For this review, take the finished solid that the model builds, in its own axes (mm). Face numbers are marked on the shaded views. A direction names the side the tool comes from. Give positions to 0.01 mm unless a question says otherwise; leave off trailing zeros. Order: outer loops, then holes, each group sorted by start corner. A loop starts at its lowest first (then second) coordinate and runs counter-clockwise, first axis right, second up. Notation, with made-up numbers: M -20,63 L 24,63 A26 ccw 24,81 Z; hole C 88,6 d9. An arc over 180 degrees is marked long. Answer as CSV lines item,"result". Start each with the question number.
1. Machinability: for the marked faces 1 and 2, which of the approach directions +Z, -Z, +X, -X, +Y, -Y give a long, thin tool a straight path to every point of the face, cutting with its end or side? Answer none if there is none.
2. For line 1 along Y through (x, z) = (36.75, 0); line 2 along X through (y, z) = (-6.75, 8.5); line 3 along Z through (x, y) = (28.5, 0.75), list the stretches that pass through material, from the lowest coordinate up.
3. Mouldability with a two-part tool opening along Y and no side actions: class the marked faces 3, 4 and 5 as pulls with the +Y half, pulls with the -Y half, needs draft (parallel to the pull), parting line crosses it, or undercut.
4. We need section D-D, the plane x = 1. Give the boundary of the cut face in (y, z), and give its area (3 significant figures).
5. We need section A-A, the plane y = 0. Give the boundary of the cut face in (x, z).
6. Clearance check with flat-ended pins moving along their axes: P1, Ø4, axis at x = 28.5, z = 7.5, coming from the -Y side; P2, Ø1.5, axis at x = -31.5, y = -3, coming from the +Z side; P3, Ø8, axis at x = -27.5, y = -5.5, coming from the +Z side. State where each tip first meets the part, or that it passes through.
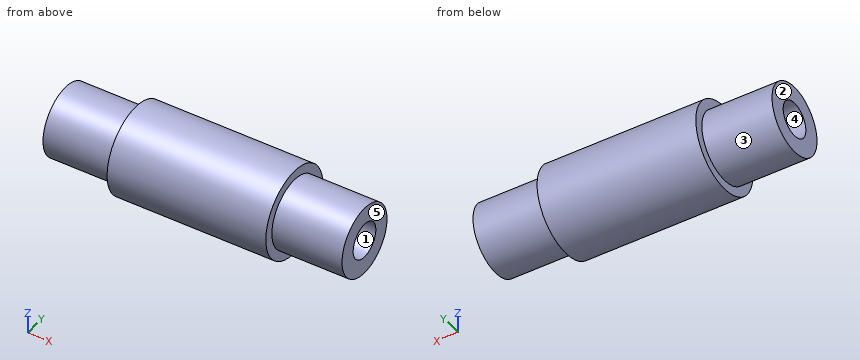
from build123d import *

# Parameters (mm, degrees)
SOCKET_1_SKETCH_W = 17.8
SOCKET_1_SKETCH_H = 4.7625
SOCKET_2_SKETCH_W = 17.8
SOCKET_2_SKETCH_H = 4.7625


with BuildPart() as part:
    # Filter_F2_T6 Sketch → Filter_F2_T6 (revolve)
    with BuildSketch(Plane.XY, mode=Mode.PRIVATE) as filter_f2_t6_sk:
        Polygon((-40.5, 0), (-40.5, 9.45), (-21.5, 9.45), (-21.5, 11.988), (21.5, 11.988), (21.5, 9.45), (40.5, 9.45), (40.5, 0), align=None)
    revolve(filter_f2_t6_sk.sketch.rotate(Axis((-1000, 0, 0), (1, 0, 0)), 90), axis=Axis((-1000, 0, 0), (1, 0, 0)))

    # Socket 1 Sketch → Socket 1 (revolve, cut)
    with BuildSketch(Plane.XY, mode=Mode.PRIVATE) as socket_1_sk:
        with Locations((-32.6, 2.38125)):
            Rectangle(SOCKET_1_SKETCH_W, SOCKET_1_SKETCH_H)
    revolve(socket_1_sk.sketch.rotate(Axis((-1000, 0, 0), (1, 0, 0)), 90), axis=Axis((-1000, 0, 0), (1, 0, 0)), mode=Mode.SUBTRACT)

    # Socket 2 Sketch → Socket 2 (revolve, cut)
    with BuildSketch(Plane.XY, mode=Mode.PRIVATE) as socket_2_sk:
        with Locations((32.6, 2.38125)):
            Rectangle(SOCKET_2_SKETCH_W, SOCKET_2_SKETCH_H)
    revolve(socket_2_sk.sketch.rotate(Axis((-1000, 0, 0), (1, 0, 0)), 90), axis=Axis((-1000, 0, 0), (1, 0, 0)), mode=Mode.SUBTRACT)


solid = part.part
Result set:
1,face 1,"+X"
1,face 2,"+Z, -Z, -X, +Y, -Y"
2,line 1,"-9.45 to -4.76, 4.76 to 9.45"
2,line 2,"-21.5 to 21.5"
2,line 3,"-9.42 to -4.7, 4.7 to 9.42"
3,face 3,"parting line crosses it"
3,face 4,"undercut"
3,face 5,"needs draft"
4,outline,"C 0,0 d23.98"
4,area,"451 mm2"
5,outline,"M -40.5,-9.45 L -21.5,-9.45 L -21.5,-11.99 L 21.5,-11.99 L 21.5,-9.45 L 40.5,-9.45 L 40.5,-4.76 L 23.7,-4.76 L 23.7,4.76 L 40.5,4.76 L 40.5,9.45 L 21.5,9.45 L 21.5,11.99 L -21.5,11.99 L -21.5,9.45 L -40.5,9.45 L -40.5,4.76 L -23.7,4.76 L -23.7,-4.76 L -40.5,-4.76 Z"
6,P1,"y = -7.68"
6,P2,"z = 9.18"
6,P3,"z = 9.33"
